Could you check a few things on this model? Use its own coordinates, in mm. A direction names the side the tool comes from. Coordinates: 2 decimals unless noted, no trailing zeros. Write each loop counter-clockwise with the first axis right and the second up, starting at its lowest first coordinate (ties: lowest second). Pieces come first, ordered by that corner, then holes.
Item 1: I want a section at B-B on y = -186.5. Please give me the cut outline in (x, z), then the cut area to 3 significant figures.
Item 2: For P1, Ø3, axis at x = -0.5, y = -250, coming from the +Z side; P2, Ø4.5, axis at y = -208.9, z = 128.24, coming from the +X side, each with a flat end and sliding along its axis, tell me the tip position at first contact or that it passes through.
Item 3: I want a section at A-A on x = -1.25. State how many separate pieces and enclosed holes the cut face has, then the cut area to 3 significant figures.
Item 4: Which directions (+Z, -Z, +X, -X, +Y, -Y) give clear straight access to the entire face, cutting with the end or side of a thin tool? Please do faces 1 (the flat face through (0, -221, 174.797)), 2 (the flat face through (0, -480, 174.797)), 3 (the flat face through (0, -481, 294.797)).
Item 5: I want a section at C-C on z = 207.5. Please give me the cut outline in (x, y).
Item 6: If I drill on probe 1 along Z at (x, y) = (-0.75, -279); probe 2 along Y at (x, z) = (4, 140); probe 3 along Y at (x, z) = (4, 220), over which ranges is the centre line in solid material (lowest first)?
from build123d import *

# Parameters (mm, degrees)
SALIENTE_EXTRUIR1_DEPTH = 4.5
CROQUIS4_R              = 18
CROQUIS4_R_2            = 2
CORTAR_EXTRUIR3_DEPTH   = 599.217436148
CHAFL_N1_SIZE           = 0.5
CROQUIS5_R              = 8
CROQUIS5_R_2            = 3
CORTAR_EXTRUIR4_DEPTH   = 599.217436148
CHAFL_N2_SIZE           = 0.5
CROQUIS3_R              = 3
CORTAR_EXTRUIR2_DEPTH   = 599.217436148
CHAFL_N3_SIZE           = 0.5
CROQUIS2_R              = 2
CORTAR_EXTRUIR1_DEPTH   = 599.217436148
CHAFL_N4_SIZE           = 0.5
CHAFL_N5_SIZE           = 0.5


with BuildPart() as part:
    # Croquis1 → Saliente-Extruir1 (new, symmetric)
    with BuildSketch(Plane(origin=(0, 0, 0), x_dir=(0, 0, -1), z_dir=(1, 0, 0))):
        Polygon((-294.796624044, -440.459461787), (-174.796624044, -290.459461787), (-174.796624044, -150.459461787), (-114.796624044, -150.459461787), (-114.796624044, -350.459461787), (-174.796624044, -440.459461787), (-174.796624044, -520.459461787), (-294.796624044, -520.459461787), align=None)
    extrude(amount=SALIENTE_EXTRUIR1_DEPTH, both=True)

    # Croquis4 → Cortar-Extruir3 (cut, through all)
    with BuildSketch(Plane(origin=(4.5, 0, 0), x_dir=(0, 0, -1), z_dir=(1, 0, 0))):
        with Locations((-143.796624044, -224.459461787)):
            Circle(CROQUIS4_R)
        with Locations((-159.35297323, -208.903112601)):
            Circle(CROQUIS4_R_2)
        with Locations((-128.240274858, -208.903112601)):
            Circle(CROQUIS4_R_2)
        with Locations((-128.240274858, -240.015810973)):
            Circle(CROQUIS4_R_2)
        with Locations((-159.35297323, -240.015810973)):
            Circle(CROQUIS4_R_2)
    extrude(amount=-CORTAR_EXTRUIR3_DEPTH, mode=Mode.SUBTRACT)

    # Chaflán1
    chafl_n1_edges = [part.edges().sort_by_distance(p)[0] for p in [
        (4.5, -224.459461787, 161.796624044),
        (4.5, -208.903112601, 161.35297323),
        (4.5, -208.903112601, 130.240274858),
        (4.5, -240.015810973, 130.240274858),
        (4.5, -240.015810973, 161.35297323),
    ]]
    chamfer(chafl_n1_edges, length=CHAFL_N1_SIZE)

    # Croquis5 → Cortar-Extruir4 (cut, through all)
    with BuildSketch(Plane(origin=(4.5, 0, 0), x_dir=(0, 0, -1), z_dir=(1, 0, 0))):
        with Locations((-144.796624044, -170.459461787)):
            Circle(CROQUIS5_R)
        with Locations((-144.796624044, -278.459461787)):
            Circle(CROQUIS5_R)
        with Locations((-124.796624044, -170.459461787)):
            Circle(CROQUIS5_R_2)
        with Locations((-164.796624044, -170.459461787)):
            Circle(CROQUIS5_R_2)
        with Locations((-164.796624044, -278.459461787)):
            Circle(CROQUIS5_R_2)
        with Locations((-124.796624044, -278.459461787)):
            Circle(CROQUIS5_R_2)
    extrude(amount=-CORTAR_EXTRUIR4_DEPTH, mode=Mode.SUBTRACT)

    # Chaflán2
    chafl_n2_edges = [part.edges().sort_by_distance(p)[0] for p in [
        (4.5, -170.459461787, 152.796624044),
        (4.5, -278.459461787, 152.796624044),
        (4.5, -170.459461787, 127.796624044),
        (4.5, -170.459461787, 167.796624044),
        (4.5, -278.459461787, 167.796624044),
        (4.5, -278.459461787, 127.796624044),
    ]]
    chamfer(chafl_n2_edges, length=CHAFL_N2_SIZE)

    # Croquis3 → Cortar-Extruir2 (cut, through all)
    with BuildSketch(Plane(origin=(4.5, 0, 0), x_dir=(0, 0, -1), z_dir=(1, 0, 0))):
        with Locations((-289.796624044, -473.459461787)):
            Circle(CROQUIS3_R)
        with Locations((-289.796624044, -513.459461787)):
            Circle(CROQUIS3_R)
        with Locations((-249.796624044, -473.459461787)):
            Circle(CROQUIS3_R)
        with Locations((-249.796624044, -513.459461787)):
            Circle(CROQUIS3_R)
        with Locations(Location((-219.796624044, -513.459461787, 0), (0, 0, 180))):
            Circle(CROQUIS3_R)
        with Locations(Location((-219.796624044, -473.459461787, 0), (0, 0, 180))):
            Circle(CROQUIS3_R)
        with Locations(Location((-179.796624044, -513.459461787, 0), (0, 0, 180))):
            Circle(CROQUIS3_R)
        with Locations(Location((-179.796624044, -473.459461787, 0), (0, 0, 180))):
            Circle(CROQUIS3_R)
    extrude(amount=-CORTAR_EXTRUIR2_DEPTH, mode=Mode.SUBTRACT)

    # Chaflán3
    chafl_n3_edges = [part.edges().sort_by_distance(p)[0] for p in [
        (4.5, -473.459461787, 292.796624044),
        (4.5, -513.459461787, 292.796624044),
        (4.5, -473.459461787, 252.796624044),
        (4.5, -513.459461787, 252.796624044),
        (4.5, -513.459461787, 216.796624044),
        (4.5, -473.459461787, 216.796624044),
        (4.5, -513.459461787, 176.796624044),
        (4.5, -473.459461787, 176.796624044),
    ]]
    chamfer(chafl_n3_edges, length=CHAFL_N3_SIZE)

    # Croquis2 → Cortar-Extruir1 (cut, through all)
    with BuildSketch(Plane(origin=(4.5, 0, 0), x_dir=(0, 0, -1), z_dir=(1, 0, 0))):
        with Locations((-234.796624044, -460.459461787)):
            Circle(CROQUIS2_R)
        with Locations((-269.796624044, -460.459461787)):
            Circle(CROQUIS2_R)
        with Locations((-199.796624044, -460.459461787)):
            Circle(CROQUIS2_R)
    extrude(amount=-CORTAR_EXTRUIR1_DEPTH, mode=Mode.SUBTRACT)

    # Chaflán4
    chafl_n4_edges = [part.edges().sort_by_distance(p)[0] for p in [
        (4.5, -460.459461787, 236.796624044),
        (4.5, -460.459461787, 271.796624044),
        (4.5, -460.459461787, 201.796624044),
    ]]
    chamfer(chafl_n4_edges, length=CHAFL_N4_SIZE)

    # Chaflán5
    chafl_n5_edges = [part.edges().sort_by_distance(p)[0] for p in [
        (-4.5, -224.459461787, 161.796624044),
        (-4.5, -170.459461787, 152.796624044),
        (-4.5, -278.459461787, 152.796624044),
    ]]
    chamfer(chafl_n5_edges, length=CHAFL_N5_SIZE)


solid = part.part
Response values:
1. outline: (-4.5, 114.8) - (4.5, 114.8) - (4.5, 174.8) - (-4.5, 174.8) - close
1. area: 540 mm2
2. P1: stops at z = 174.8
2. P2: stops at x = 4.25
3. separate pieces: 1
3. enclosed holes: 22
3. area: 31,500 mm2
4. face 1: +Z, +X, -X, +Y
4. face 2: -Z, +X, -X, -Y
4. face 3: +Z, +X, -X, +Y, -Y
5. outline: (-4.5, -520.46) - (4.5, -520.46) - (4.5, -331.34) - (-4.5, -331.34) - close
6. probe 1: z = 114.8 to 121.85, 127.75 to 136.81, 152.78 to 161.85, 167.75 to 174.8
6. probe 2: y = -388.26 to -284.86, -272.06 to -242.05, -206.86 to -176.86, -164.06 to -150.46
6. probe 3: y = -520.46 to -516.45, -510.47 to -476.45, -470.47 to -346.96
